The listing builds one solid part. Answer for the finished solid, in the listing's coordinates (mm). Coordinates: 2 decimals unless noted, no trailing zeros. Loops run counter-clockwise (first coordinate to the right, second up) from the corner with the lowest first, then second, coordinate; pieces in that order, holes last. Notation, with made-up numbers: M 6.5,12 L 60.5,12 A25 ccw 60.5,41 Z; hole C 43.5,60.5 d3. An arc over 180 degrees is marked long. Answer as a JSON object with one key per item and string values. Group by question number.
1. Given pin 1 (1 mm diameter, centred on x = 275, y = 5, fed in from -Z); pin 2 (4 mm diameter, centred on x = 157.5, y = -8.5, fed in from +Z); pin 3 (5 mm diameter, centred on x = 422, y = 6, fed in from +Z); pin 4 (10 mm diameter, centred on x = 364.5, z = -17.5, fed in from +Y), each flat-ended and moving along its own axis, determine where each tip first touches the part or whether it passes through.
2. Straight lines are drawn through the part: L1, parallel to X at y = 0.25, z = -7.5; L2, parallel to X at y = 3.5, z = -16; L3, parallel to Y at x = 306, z = 1. For each, find the intervals that lie inside material, in ascending order.
3. A cutting plane is placed at A-A on x = 429.5. Give the vertices of the cut face in (y, z).
from build123d import *

# Parameters (mm, degrees)
SALIENTE_EXTRUIR1_DEPTH = 480
REDONDEO1_R             = 10
CROQUIS2_R              = 3
CORTAR_EXTRUIR1_DEPTH   = 25


with BuildPart() as part:
    # Croquis1 → Saliente-Extruir1 (new body)
    with BuildSketch(Plane(origin=(0, 0, 0), x_dir=(0, 0, -1), z_dir=(1, 0, 0))):
        with BuildLine():
            Line((0, 12.5), (15, 12.5))
            ThreePointArc((15, 12.5), (27.5, 0), (15, -12.5))
            Line((15, -12.5), (0, -12.5))
            ThreePointArc((0, -12.5), (-12.5, 0), (0, 12.5))
        make_face()
    extrude(amount=SALIENTE_EXTRUIR1_DEPTH)

    # Redondeo1
    redondeo1_edges = [part.edges().sort_by_distance(p)[0] for p in [
        (480, 0, -27.5),
        (480, 12.5, -7.5),
        (480, 0, 12.5),
        (480, -12.5, -7.5),
    ]]
    fillet(redondeo1_edges, radius=REDONDEO1_R)

    # Croquis2 → Cortar-Extruir1 (cut)
    with BuildSketch(Plane(origin=(0, 12.5, 0), x_dir=(1, 0, 0), z_dir=(0, 1, 0))):
        with Locations((32, 7.5)):
            Circle(CROQUIS2_R)
    extrude(amount=-CORTAR_EXTRUIR1_DEPTH, mode=Mode.SUBTRACT)


solid = part.part
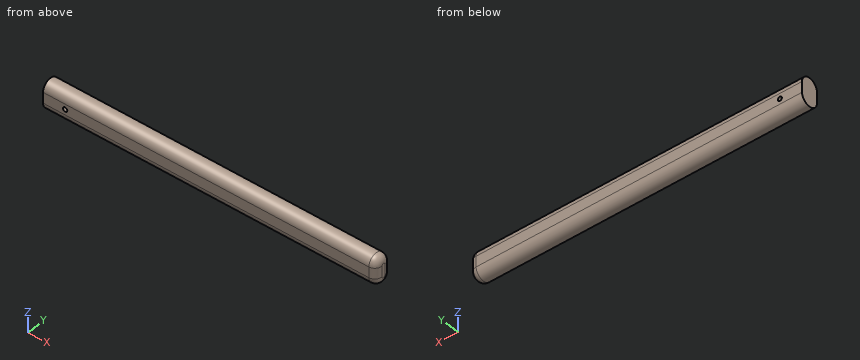
From the geometry:
{
 "1": {"pin 1": "stops at z = -26.66", "pin 2": "stops at z = 10.68", "pin 3": "stops at z = 12", "pin 4": "stops at y = 12.5"},
 "2": {"L1": "x = 0 to 29, 35 to 480", "L2": "x = 0 to 479.93", "L3": "y = -12.46 to 12.46"},
 "3": {"outline": "M -12.5,-15 A12.5 ccw 12.5,-15 L 12.5,0 A12.5 ccw -12.5,0 Z"}
}
